For this review, take the finished solid that the model builds, in its own axes (mm). Coordinates: 2 decimals unless noted, no trailing zeros. Loops run counter-clockwise (first coordinate to the right, second up) from the corner with the lowest first, then second, coordinate; pieces in that order, holes last. Notation, with made-up numbers: M 52.25,-38.75 L 102.25,-38.75 A18 cw 102.25,-13.75 Z; hole C 41.5,23.25 d8. An arc over 180 degrees is marked long. Put each result on its own line as item: value.
```python
from build123d import *
from build123d.topology import SkipClean

# Parameters (mm, degrees)
SKETCH1_R                = 4.5
MAIN_BASE_DEPTH          = 3
BOSS_EXTRUDE1_DEPTH      = 0.5
BOSS_EXTRUDE1_DEPTH_BACK = 0.5
SKETCH5_W                = 0.4
SKETCH5_H                = 2
SKETCH5_H_2              = 2.5


with BuildPart() as part:
    # Sketch1 → main_base (new body)
    with BuildSketch(Plane.XY):
        Circle(SKETCH1_R)
    extrude(amount=MAIN_BASE_DEPTH)

    # Sketch2 → pulley_cut_out (revolve, cut)
    with BuildSketch(Plane(origin=(0, 0, 0), x_dir=(0, 0, -1), z_dir=(1, 0, 0)), mode=Mode.PRIVATE) as pulley_cut_out_sk:
        Polygon((-2.5, 4.5), (-0.5, 4.5), (-1, 4), (-2, 4), align=None)
    revolve(pulley_cut_out_sk.sketch.rotate(Axis((0, 0, 0), (0, 0, 1)), 90), axis=Axis((0, 0, 0), (0, 0, 1)), mode=Mode.SUBTRACT)

    # Sketch4 → rotating_point (revolve)
    with SkipClean():  # the faces are left unmerged after this step: merging them gives an invalid solid
        with BuildSketch(Plane(origin=(0, 0, 0), x_dir=(1, 0, 0), z_dir=(0, 1, 0))):
            with BuildLine():
                ThreePointArc((0, 1), (-0.707106781, 0.707106781), (-1, 0))
                Line((-1, 0), (0, 0))
                Line((0, 0), (0, 1))
            make_face()
            with BuildLine():
                Line((0, 1), (0, 0))
                Line((0, 0), (1, 0))
                ThreePointArc((1, 0), (0.707106781, 0.707106781), (0, 1))
            make_face()
            with BuildLine():
                Line((1, -3), (0, -3))
                Line((0, -3), (0, -4))
                ThreePointArc((0, -4), (0.707106781, -3.707106781), (1, -3))
            make_face()
            with BuildLine():
                Line((0, -4), (0, -3))
                Line((0, -3), (-1, -3))
                ThreePointArc((-1, -3), (-0.707106781, -3.707106781), (0, -4))
            make_face()
        revolve(axis=Axis((0, 0, -1), (0, 0, 1)))
    add(part.part.scale(1), mode=Mode.REPLACE)  # the faces are merged on a copy

    # Sketch5 → Boss-Extrude1 (add, two sides: drawn at the far end of the back side and taken through both)
    with BuildSketch(Plane(origin=(0, 0, 0), x_dir=(0, 0, -1), z_dir=(1, 0, 0)).offset(-BOSS_EXTRUDE1_DEPTH_BACK)):
        with Locations((-2.75, 5)):
            Rectangle(SKETCH5_W, SKETCH5_H)
        with Locations((-1.75, 4.75)):
            Rectangle(SKETCH5_W, SKETCH5_H_2)
    extrude(amount=BOSS_EXTRUDE1_DEPTH + BOSS_EXTRUDE1_DEPTH_BACK)


solid = part.part
```
(1) Draft analysis for pull direction Z (two halves, no side actions). For faces 1 (the cylindrical face through (0.867, 3.905, 1.507)), 2 (the flat face through (0, 5, 2.55)), 3 (the flat face through (1, -1, 3)), 4 (the cylindrical face through (-0.59, 4.46, 0.25)), state which applies: +Z half, -Z half, draft (parallel to the pull), parting line (faces both ways), or undercut.
Determined:
face 1: undercut
face 2: undercut
face 3: +Z half
face 4: draft
(2) Add section A-A (y = 0). Write out the cut boundary in (x, z), plus the area to 3 significant figures.
Determined:
outline: M -4.5,0 L -1,0 A1 ccw 1,0 L 4.5,0 L 4.5,0.5 L 4,1 L 4,2 L 4.5,2.5 L 4.5,3 L 1,3 A1 ccw -1,3 L -4.5,3 L -4.5,2.5 L -4,2 L -4,1 L -4.5,0.5 Z
area: 28.6 mm^2
(3) Add section D-D (z = 0.7). Write out the cut boundary in (x, y), plus the area to 3 significant figures.
Determined:
outline: C 0,0 d8.6
area: 58.1 mm^2
(4) For pin 1 (1.1 mm diameter, centred on x = 0, y = 5.5, fed in from -Z); pin 2 (2 mm diameter, centred on y = 2, z = 3, fed in from -X); pin 3 (3 mm diameter, centred on x = -3, y = 5, fed in from -Z), all flat-tipped, find the tip position at first contact; note any pin that passes through.
Determined:
pin 1: stops at z = 1.55
pin 2: stops at x = -4.39
pin 3: stops at z = 0
(5) Add section C-C (z = 2.75). Write out the cut boundary in (x, y), plus the area to 3 significant figures.
Determined:
outline: M -0.5,4.47 A4.5 ccw long 0.5,4.47 L 0.5,6 L -0.5,6 Z
area: 65.1 mm^2
(6) Wall thickness on line 1 along Z through (x, y) = (2, -1.75); line 2 along Z through (x, y) = (4, 1.25); line 3 along Y through (x, z) = (2.5, 0.15): over which ranges is each line inside the solid? List them lowest first. Write a range as [from, to].
Determined:
line 1: z = [0, 3]
line 2: z = [0, 0.81], [2.19, 3]
line 3: y = [-3.74, 3.74]
(7) Add section B-B (x = 0). Write out the cut boundary in (y, z).
Determined:
outline: M -4.5,0 L -1,0 A1 ccw 1,0 L 4.5,0 L 4.5,0.5 L 4,1 L 4,1.55 L 6,1.55 L 6,1.95 L 4,1.95 L 4,2 L 4.5,2.5 L 4.5,2.55 L 6,2.55 L 6,2.95 L 4.5,2.95 L 4.5,3 L 1,3 A1 ccw -1,3 L -4.5,3 L -4.5,2.5 L -4,2 L -4,1 L -4.5,0.5 Z
